Part model, mm, in its own coordinate system. Round coordinates to 2 decimals unless told otherwise and drop trailing zeros. Write each loop counter-clockwise with the first axis right and the second up, starting at its lowest first coordinate (ties: lowest second). Pieces come first, ordered by that corner, then holes.
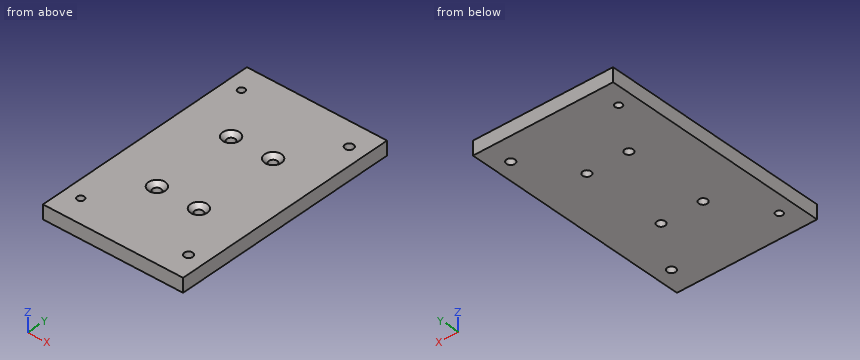
```python
from build123d import *

# Parameters (mm, degrees)
F0_W           = 100
F0_H           = 165
F0_R           = 2.5
F0_R_2         = 3
F1_DEPTH       = 10
F2_D           = 6
F2_CSINK_D     = 12
F2_CSINK_ANGLE = 90
F3_D           = 6


with BuildPart() as f1:
    # F0 (on Top) → F1 (new body)
    with BuildSketch(Plane.XY):
        Rectangle(F0_W, F0_H)
        with Locations((-38.5, -65)):
            Circle(F0_R, mode=Mode.SUBTRACT)
        with Locations((-15, -30)):
            Circle(F0_R_2, mode=Mode.SUBTRACT)
        with Locations((38.5, -65)):
            Circle(F0_R, mode=Mode.SUBTRACT)
        with Locations((15, -30)):
            Circle(F0_R_2, mode=Mode.SUBTRACT)
        with Locations((-15, 30)):
            Circle(F0_R_2, mode=Mode.SUBTRACT)
        with Locations((-38.5, 65)):
            Circle(F0_R, mode=Mode.SUBTRACT)
        with Locations((15, 30)):
            Circle(F0_R_2, mode=Mode.SUBTRACT)
        with Locations((38.5, 65)):
            Circle(F0_R, mode=Mode.SUBTRACT)
        with Locations((-15, 30)):
            Circle(F0_R_2)
        with Locations((-15, -30)):
            Circle(F0_R_2)
        with Locations((15, -30)):
            Circle(F0_R_2)
        with Locations((38.5, -65)):
            Circle(F0_R)
        with Locations((15, 30)):
            Circle(F0_R_2)
        with Locations((38.5, 65)):
            Circle(F0_R)
    extrude(amount=-F1_DEPTH)

    # F2 (through all)
    with Locations(Plane.XY):
        with Locations((-15, 30), (15, 30), (-15, -30), (15, -30)):
            CounterSinkHole(F2_D / 2, F2_CSINK_D / 2, counter_sink_angle=F2_CSINK_ANGLE)

    # F3 (through all)
    with Locations(Plane.XY):
        with Locations((38.5, 65), (38.5, -65)):
            Hole(F3_D / 2)


solid = f1.part
```
Q1. Cut at A-A on y = -65. Write the cut outline in (x, z).
Values follow:
outline: (-50, -10) - (-41, -10) - (-41, 0) - (-50, 0) - close; (-36, -10) - (35.5, -10) - (35.5, 0) - (-36, 0) - close; (41.5, -10) - (50, -10) - (50, 0) - (41.5, 0) - close
Q2. Cut at C-C on z = -1.5. State how many separate pieces and enclosed holes the cut face has, plus the area to 3 significant figures.
Values follow:
separate pieces: 1
enclosed holes: 8
area: 16,100 mm2
Q3. Cut at B-B on x = -38.5. Write the cut outline in (y, z), plus the area to 3 significant figures.
Values follow:
outline: (-82.5, -10) - (-67.5, -10) - (-67.5, 0) - (-82.5, 0) - close; (-62.5, -10) - (62.5, -10) - (62.5, 0) - (-62.5, 0) - close; (67.5, -10) - (82.5, -10) - (82.5, 0) - (67.5, 0) - close
area: 1,550 mm2
Q4. Wall check: L1, parallel to X at y = 30, z = -4.25; L2, parallel to Y at x = -15, z = -7.75; L3, parallel to Y at x = 38.5, z = -4. Give the ranges that are in metal, low to high.
Values follow:
L1: x = -50 to -18, -12 to 12, 18 to 50
L2: y = -82.5 to -33, -27 to 27, 33 to 82.5
L3: y = -82.5 to -68, -62 to 62, 68 to 82.5
Q5. Drop flat-ended pins along their axis: pin 1 (7 mm diameter, centred on x = 38.5, y = -65, fed in from -Z); pin 2 (8 mm diameter, centred on x = -15, y = -30, fed in from +Z). Give the stop position or say it passes through.
Values follow:
pin 1: stops at z = -10
pin 2: stops at z = -2
Q6. Cut at D-D on y = -30. Write the cut outline in (x, z), plus the area to 3 significant figures.
Values follow:
outline: (-50, -10) - (-18, -10) - (-18, -3) - (-21, 0) - (-50, 0) - close; (-12, -10) - (12, -10) - (12, -3) - (9, 0) - (-9, 0) - (-12, -3) - close; (18, -10) - (50, -10) - (50, 0) - (21, 0) - (18, -3) - close
area: 862 mm2
